Could you check a few things on this model? Use its own coordinates, in mm. Face numbers are marked on the shaded views. A direction names the side the tool comes from. Give positions to 0.01 mm unless a question says otherwise; leave off trailing zeros. Order: outer loops, then holes, each group sorted by start corner. A loop starts at its lowest first (then second) coordinate and runs counter-clockwise, first axis right, second up.
from build123d import *

# Parameters (mm, degrees)
SKETCH1_W           = 27.4
SKETCH1_H           = 6
BOSS_EXTRUDE1_DEPTH = 2
SKETCH2_W           = 1.5
SKETCH2_H           = 6
BOSS_EXTRUDE2_DEPTH = 25
SKETCH3_R           = 1.4
CUT_EXTRUDE1_DEPTH  = 39.584452828
FILLET1_R           = 3
SKETCH4_W           = 27.4
SKETCH4_H           = 2
BOSS_EXTRUDE3_DEPTH = 10
FILLET2_R           = 4


with BuildPart() as part:
    # Sketch1 → Boss-Extrude1 (new body)
    with BuildSketch(Plane.XY):
        Rectangle(SKETCH1_W, SKETCH1_H)
    extrude(amount=BOSS_EXTRUDE1_DEPTH)

    # Sketch2 → Boss-Extrude2 (add)
    with BuildSketch(Plane.XY.offset(2)):
        with Locations((-12.95, 0)):
            Rectangle(SKETCH2_W, SKETCH2_H)
        with Locations((12.95, 0)):
            Rectangle(SKETCH2_W, SKETCH2_H)
    extrude(amount=BOSS_EXTRUDE2_DEPTH)

    # Sketch3 → Cut-Extrude1 (cut, through all)
    with BuildSketch(Plane(origin=(13.7, 0, 0), x_dir=(0, 0, -1), z_dir=(1, 0, 0))):
        with Locations((-24.1, 0)):
            Circle(SKETCH3_R)
    extrude(amount=-CUT_EXTRUDE1_DEPTH, mode=Mode.SUBTRACT)

    # Fillet1
    fillet1_edges = [part.edges().sort_by_distance(p)[0] for p in [
        (-12.95, -3, 27),
        (12.95, -3, 27),
        (-12.95, 3, 27),
        (12.95, 3, 27),
    ]]
    fillet(fillet1_edges, radius=FILLET1_R - 0.0001)  # a hair under: the kernel refuses the full size

    # Sketch4 → Boss-Extrude3 (add)
    with BuildSketch(Plane(origin=(0, 3, 0), x_dir=(1, 0, 0), z_dir=(0, 1, 0))):
        with Locations((0, -1)):
            Rectangle(SKETCH4_W, SKETCH4_H)
    extrude(amount=BOSS_EXTRUDE3_DEPTH)

    # Fillet2
    fillet2_edges = [part.edges().sort_by_distance(p)[0] for p in [
        (12.2, 0, 2),
        (-12.2, 0, 2),
    ]]
    fillet(fillet2_edges, radius=FILLET2_R)


solid = part.part
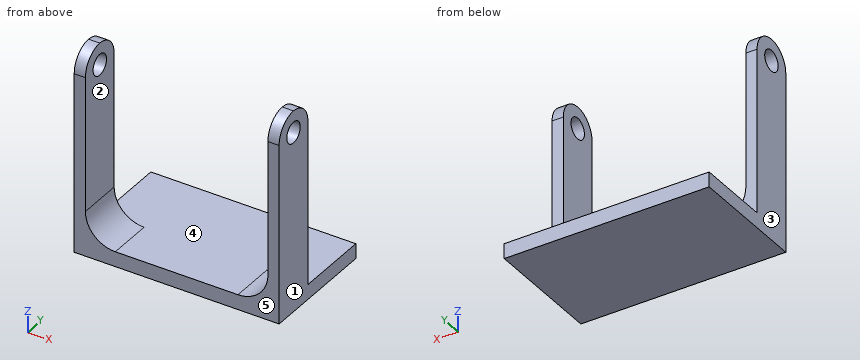
Item 1: Imagine slicing it at A-A on z = 14.25. List the corners of the cut face in (x, y) for me.
Findings:
outline: (-13.7, -3) - (-12.2, -3) - (-12.2, 3) - (-13.7, 3) - close; (12.2, -3) - (13.7, -3) - (13.7, 3) - (12.2, 3) - close
Item 2: Imagine slicing it at D-D on x = 4. List the corners of the cut face in (y, z) for me.
Findings:
outline: (-3, 0) - (13, 0) - (13, 2) - (-3, 2) - close
Item 3: For the marked faces 1 and 2, which set-ups out of +Z, -Z, +X, -X, +Y, -Y let a thin tool reach every point of the face, with its end or its side?
Findings:
face 1: +Z, -Z, +X, +Y, -Y
face 2: +Z, +Y, -Y
Item 4: For pin 1 (1.6 mm diameter, centred on x = -12, z = 16.5, fed in from +Y); pin 2 (1.5 mm diameter, centred on x = 5.5, y = 5, fed in from +Z), each with a flat end and sliding along its axis, tell me the tip position at first contact or that it passes through.
Findings:
pin 1: stops at y = 3
pin 2: stops at z = 2
Item 5: Please list where these lines run through material, in increasing order: line 1 along Y through (x, z) = (-13.3, 24.1); line 2 along X through (y, z) = (0.5, 16.5); line 3 along Z through (x, y) = (-11.5, 7).
Findings:
line 1: y = -3 to -1.4, 1.4 to 3
line 2: x = -13.7 to -12.2, 12.2 to 13.7
line 3: z = 0 to 2
Item 6: Imagine slicing it at B-B on x = -11.5. List the corners of the cut face in (y, z) for me.
Findings:
outline: (-3, 0) - (13, 0) - (13, 2) - (3, 2) - (3, 3.74) - (-3, 3.74) - close
Item 7: We'd pull the mould along X, two halves only. Please class the marked faces 3, 4 and 5: +X half, -X half, draft (parallel to the pull), parting line (faces both ways), or undercut.
Findings:
face 3: -X half
face 4: undercut
face 5: draft
Item 8: Imagine slicing it at C-C on y = 7.25. List the corners of the cut face in (x, z) for me.
Findings:
outline: (-13.7, 0) - (13.7, 0) - (13.7, 2) - (-13.7, 2) - close
